Verification items for the finished model (mm, model axes). Coordinates: 2 decimals unless noted, no trailing zeros. Order: outer loops, then holes, each group sorted by start corner. A loop starts at its lowest first (then second) coordinate and runs counter-clockwise, first axis right, second up. Notation, with made-up numbers: (-37.5, 7.25) -> (7.5, 7.25) arc R23 ccw to (7.5, 22.25) -> close; hole circle Ø4 at (63, -7). An arc over 180 degrees is marked (long way). Use CSV: the item, a comma, the result in double quotes. Start each with the question number.
1) Scan lines: line 1 along X through (y, z) = (44, 49); line 2 along Z through (x, y) = (64, 13); line 3 along X through (y, z) = (11, 13). Record each from-to range of solid material in increasing order.
2) Sectioned sample at B-B on x = 61.5. Record the boundary of the cut face in (y, z), then the cut area to 3 significant figures.
3) Sectioned sample at A-A on z = 13.5. Record the boundary of the cut face in (x, y), then the cut area to 3 significant figures.
4) Release check for a two-part mould opening along Y. For faces 1 (the flat face through (62, 45, 101.6)), 2 (the flat face through (-76.2, 45, 63)), 3 (the flat face through (1, 0, 63)), 4 (the cylindrical face through (38.11, 43.56, 50.09)) record: released by +Y, released by -Y, zero draft, split by the parting line, or undercut.
5) Sectioned sample at C-C on y = 41. Record the boundary of the cut face in (x, z).
6) Sectioned sample at D-D on x = 45.5. Record the boundary of the cut face in (y, z).
Autodesk Inventor part; units mm, degrees
ref_plane "YZ Plane" through (0, 0, 0) normal (1, 0, 0) x (0, 1, 0)
ref_plane "XZ Plane" through (0, 0, 0) normal (0, 1, 0) x (-1, 0, 0)
ref_plane "XY Plane" through (0, 0, 0) normal (0, 0, 1) x (1, 0, 0)
sketch "Sketch1" plane through (0, 0, 0) normal (0, 0, 1) x (1, 0, 0)
  line L0 (0, 0) -> (76.2, 0)
  line L1 (76.2, 0) -> (76.2, 88.9)
  line L2 (76.2, 88.9) -> (0, 88.9)
  line L3 (0, 88.9) -> (0, 0)
  dimension "d0" = 76.2
  dimension "d1" = 88.9
extrude "Extrusion1" add sketch "Sketch1" along normal blind 127
sketch "Sketch3" plane through (0, 0, 0) normal (0, 0, -1) x (-1, 0, 0)
  circle A0 centre (-82.55, 44.45) radius 44.45
  dimension "d4" = 88.9
extrude "Extrusion2" cut sketch "Sketch3" against normal blind 101.6
sketch "Sketch4" plane through (0, 0, 0) normal (-1, 0, 0) x (0, 0, 1)
  line L0 (0, 0) -> (127, 0)
  line L1 (127, 0) -> (127, 88.9)
  line L2 (127, 88.9) -> (0, 88.9)
  line L3 (0, 88.9) -> (0, 0)
extrude "Extrusion3" add sketch "Sketch4" along normal blind 76.2
sketch "Sketch5" plane through (76.2, 0, 0) normal (0, -1, 0) x (1, 0, 0)
  line L0 (-152.4, 0) -> (0, 0)
  line L1 (0, 0) -> (0, 127)
  line L2 (0, 127) -> (-152.4, 127)
  line L3 (-152.4, 0) -> (-152.4, 127)
  line L4 (0, 63.5) -> (-88.9, 63.5)
  point P0 (-76.2, 0)
  dimension "d9" = 88.9
sketch "Sketch6" plane through (76.2, 88.9, 127) normal (0, 1, 0) x (1, 0, 0)
  line L0 (0, 127) -> (-152.4, 127)
  line L1 (-152.4, 0) -> (-152.4, 127)
  line L2 (0, 0) -> (-152.4, 0)
  line L3 (0, 127) -> (0, 0)
  line L4 (0, 127) -> (0, 63.5)
  line L5 (0, 63.5) -> (-88.9, 63.5)
  point P0 (-76.2, 127)
  dimension "d10" = 63.5
  dimension "d11" = 88.9
properties part number "Holder"
Answers follow:
1,line 1,"x = -76.2 to 38.1"
1,line 2,"z = 101.6 to 127"
1,line 3,"x = -76.2 to 53.28"
2,outline,"(0, 0) -> (5.3, 0) -> (5.3, 101.6) -> (83.6, 101.6) -> (83.6, 0) -> (88.9, 0) -> (88.9, 127) -> (0, 127) -> close"
2,area,"3,340 mm²"
3,outline,"(-76.2, 0) -> (76.2, 0) -> (76.2, 0.46) arc R44.45 cw to (76.2, 88.44) -> (76.2, 88.9) -> (-76.2, 88.9) -> close"
3,area,"11,000 mm²"
4,face 1,"undercut"
4,face 2,"zero draft"
4,face 3,"released by -Y"
4,face 4,"undercut"
5,outline,"(-76.2, 0) -> (38.23, 0) -> (38.23, 101.6) -> (76.2, 101.6) -> (76.2, 127) -> (-76.2, 127) -> close"
6,outline,"(0, 0) -> (19.89, 0) -> (19.89, 101.6) -> (69.01, 101.6) -> (69.01, 0) -> (88.9, 0) -> (88.9, 127) -> (0, 127) -> close"
